from build123d import *

# Parameters (mm, degrees)
F0_W     = 111.369263
F0_H     = 66.945155
F1_DEPTH = 15
F2_R     = 14.959389
F3_DEPTH = 25
F4_R     = 5


with BuildPart() as f1:
    # F0 (on Front) → F1 (new body)
    with BuildSketch(Plane.XZ):
        with Locations((-1.347209, 4.700554)):
            Rectangle(F0_W, F0_H)
    extrude(amount=F1_DEPTH)

    # F2 (on face) → F3 (join)
    with BuildSketch(Plane.XZ.offset(15)):
        with Locations((8.211179, 10.319434)):
            Circle(F2_R)
    extrude(amount=F3_DEPTH)

    # F4
    f4_edges = [f1.edges().sort_by_distance(p)[0] for p in [
        (54.337423, -7.5, 38.173132),
        (54.337423, -7.5, -28.772023),
        (-6.74821, -40, 10.319434),
    ]]
    fillet(f4_edges, radius=F4_R)


solid = f1.part
Build history of the part. All positions in model axes, mm. A direction names the side the tool comes from. Round coordinates to 2 decimals unless told otherwise and drop trailing zeros. Loops run counter-clockwise (first coordinate to the right, second up) from the corner with the lowest first, then second, coordinate; pieces in that order, holes last. Notation, with made-up numbers: (25.25, -32.5) -> (46.25, -32.5) arc R25 cw to (46.25, -5.5) -> close; hole circle Ø5 at (50, 31). An arc over 180 degrees is marked (long way). One line per item, written item: value. Start each with the question number.
Q1. 3-axis set-ups, long thin cutter, end or side, ignore diameter. For faces 1 (the face through (52.83, -7.6, -27.35)), 2 (the face through (22.48, -24.86, 14.81)): which of +Z, -Z, +X, -X, +Y, -Y reach the whole face in a straight line?
Q2. Probe line 1 along Y through (x, z) = (48.5, -9); line 2 along Z through (x, y) = (4.5, -29); line 3 along X through (y, z) = (-33.5, 5.5). List the from-to ranges inside material, lowest first.
Q3. Cut at A-A on x = -43. List the corners of the cut face in (y, z), plus the area to 3 significant figures.
Q4. Drop flat-ended pins along their axis: pin 1 Ø12 at (x, z) = (-40.5, -3) entering from -Y; pin 2 Ø4 at (x, y) = (7, -18.5) entering from -Z. Give the stop position or say it passes through.
Q5. Cut at C-C on y = -29.5. List the corners of the cut face in (x, z), plus the area to 3 significant figures.
Q6. Cut at B-B on z = 31. List the corners of the cut face in (x, y), plus the area to 3 significant figures.
Computed:
1. face 1: -Z, +X, +Y, -Y
1. face 2: -Y
2. line 1: -15 to 0
2. line 2: -4.17 to 24.81
2. line 3: -5.95 to 22.37
3. outline: (-15, -28.77) -> (0, -28.77) -> (0, 38.17) -> (-15, 38.17) -> close
3. area: 1,000 mm²
4. pin 1: y = -15
4. pin 2: z = -4.64
5. outline: circle Ø29.92 at (8.21, 10.32)
5. area: 703 mm²
6. outline: (-57.03, -15) -> (54.34, -15) -> (54.34, 0) -> (-57.03, 0) -> close
6. area: 1,670 mm²
